from build123d import *

# Parameters (mm, degrees)
BOSS_EXTRUDE1_DEPTH = 30
SKETCH6_W           = 15
SKETCH6_H           = 30
BOSS_EXTRUDE2_DEPTH = 24
BOSS_EXTRUDE5_DEPTH = 10
SKETCH15_R          = 1.5
BOSS_EXTRUDE7_DEPTH = 8
SKETCH7_R           = 1.5
BOSS_EXTRUDE8_DEPTH = 8


with BuildPart() as part:
    # Sketch2 → Boss-Extrude1 (new body)
    with BuildSketch(Plane.XY):
        Polygon((-35.659220441, 48.994166095), (20.212047263, 48.994166095), (3.020324726, 8.994166095), (36.417587641, -13.019984577), (36.417587641, -68.485610583), (19.225865104, -108.485610583), (33.318130441, -145.920995684), (-101.80917988, -146.898605829), (-88.260031439, -109.263242453), (-106.02870282, -69.516171603), (-106.831218915, -14.056351587), (-73.755968311, 8.438710038), (-91.524639692, 48.185780888), align=None)
    extrude(amount=BOSS_EXTRUDE1_DEPTH)

    # Sketch6 → Boss-Extrude2 (add)
    with BuildSketch(Plane(origin=(0, 0, 0), x_dir=(0, 0, -1), z_dir=(1, 0, 0))):
        with Locations((-14.441506787, -108.571370402)):
            Rectangle(SKETCH6_W, SKETCH6_H)
    extrude(amount=BOSS_EXTRUDE2_DEPTH)

    # Sketch13 → Boss-Extrude5 (add, symmetric)
    with BuildSketch(Plane(origin=(0, 0, 15), x_dir=(-1, 0, 0), z_dir=(0, 0, -1))):
        Polygon((92.491049439, -97.377625596), (87.716914543, -108.485610583), (92.491049439, -121.167856773), align=None)
    extrude(amount=BOSS_EXTRUDE5_DEPTH, both=True)

    # Sketch15 → Boss-Extrude7 (add, symmetric)
    with BuildSketch(Plane.ZY.offset(92.491049439)):
        with Locations(Location((14.163706185, -101.373718374, 0), (0, 0, 180))):
            Circle(SKETCH15_R)
        with Locations(Location((14.163706185, -118.873718374, 0), (0, 0, 180))):
            Circle(SKETCH15_R)
    extrude(amount=BOSS_EXTRUDE7_DEPTH, both=True)

    # Sketch7 → Boss-Extrude8 (add, symmetric)
    with BuildSketch(Plane(origin=(24, 0, 0), x_dir=(0, 0, -1), z_dir=(1, 0, 0))):
        with Locations((-14.163706185, -118.873718374)):
            Circle(SKETCH7_R)
        with Locations((-14.163706185, -101.373718374)):
            Circle(SKETCH7_R)
    extrude(amount=BOSS_EXTRUDE8_DEPTH, both=True)


solid = part.part
Geometry: final body of the model. Coordinates: model frame, mm. A direction names the side the tool comes from. Give positions to 0.01 mm unless a question says otherwise; leave off trailing zeros. Order: outer loops, then holes, each group sorted by start corner. A loop starts at its lowest first (then second) coordinate and runs counter-clockwise, first axis right, second up. Notation, with made-up numbers: (2, 88.5) -> (7, 88.5) arc R28 cw to (7, 119.5) -> close; hole circle Ø11 at (28.5, 49). An arc over 180 degrees is marked (long way). Answer as a JSON object with one key per item and string values.
Q1. Section D-D (x = 26.5). Output: boundary loops of the cut face in (y, z), plus the area to 3 significant figures.
Entries:
{"outline": "(-145.97, 0) -> (-127.81, 0) -> (-127.81, 30) -> (-145.97, 30) -> close; circle Ø3 at (-118.87, 14.16); circle Ø3 at (-101.37, 14.16); (-91.56, 0) -> (-6.48, 0) -> (-6.48, 30) -> (-91.56, 30) -> close", "area": "3,110 mm^2"}
Q2. Material intervals for probe 1 along X at (y, z) = (-104.5, 10.75); probe 2 along Y at (x, z) = (14, 15); probe 3 along Y at (x, z) = (17, 15.25), sorted ascending.
Entries:
{"probe 1": "x = -92.49 to 24", "probe 2": "y = -146.06 to 1.76, 34.54 to 48.99", "probe 3": "y = -146.04 to -0.22, 41.52 to 48.99"}
Q3. Section C-C (y = -114). Output: boundary loops of the cut face in (x, z).
Entries:
{"outline": "(-92.49, 5) -> (-89.97, 5) -> (-89.97, 0) -> (21.3, 0) -> (21.3, 6.94) -> (24, 6.94) -> (24, 21.94) -> (21.3, 21.94) -> (21.3, 30) -> (-89.97, 30) -> (-89.97, 25) -> (-92.49, 25) -> close"}
Q4. Draft query along Y for faces 1 (the flat face through (-8, 48.994, 15)), 2 (the flat face through (-91, -110, 5)), 3 (the flat face through (-34, -48, 30)). Return one class per face: released by +Y, released by -Y, zero draft, split by the parting line, or undercut.
Entries:
{"face 1": "released by +Y", "face 2": "undercut", "face 3": "zero draft"}
Q5. Section B-B (z = 10.5). Output: boundary loops of the cut face in (x, y), plus the area to 3 significant figures.
Entries:
{"outline": "(-106.83, -14.06) -> (-106.03, -69.52) -> (-92.49, -99.8) -> (-92.49, -121.02) -> (-101.81, -146.9) -> (33.32, -145.92) -> (24, -121.17) -> (24, -97.38) -> (36.42, -68.49) -> (36.42, -13.02) -> (3.02, 8.99) -> (20.21, 48.99) -> (-35.66, 48.99) -> (-91.52, 48.19) -> (-73.76, 8.44) -> close", "area": "23,800 mm^2"}
Q6. First-contact query: pin 1 (1.4 mm diameter, centred on x = 22, y = -105.5, fed in from -Z); pin 2 (1 mm diameter, centred on y = -42.5, z = 26, fed in from -X); pin 3 (2.5 mm diameter, centred on y = -119.5, z = 14, fed in from +X). Flat tips, straight axial feed; report the tip coordinate or a pass-through.
Entries:
{"pin 1": "stops at z = 6.94", "pin 2": "stops at x = -106.43", "pin 3": "stops at x = 32"}
Q7. Access query for faces 4 (the flat face through (-91, -110, 25)), 5 (the flat face through (23, -109, 6.942)), 6 (the flat face through (-90.53, -2.97, 14.79)). Directions: +Z, -Z, +X, -X, +Y, -Y. A direction counts if a zero-diameter tool reaches every point of the face in a straight line with its end or side. Return the directions, or none.
Entries:
{"face 4": "+Z, -X", "face 5": "-Z, +X", "face 6": "+Z, -Z, -X"}
Q8. Section A-A (x = -94.5). Output: boundary loops of the cut face in (y, z), plus the area to 3 significant figures.
Entries:
{"outline": "(-146.85, 0) -> (-126.6, 0) -> (-126.6, 30) -> (-146.85, 30) -> close; circle Ø3 at (-118.87, 14.16); circle Ø3 at (-101.37, 14.16); (-95.3, 0) -> (-5.67, 0) -> (-5.67, 30) -> (-95.3, 30) -> close", "area": "3,310 mm^2"}
